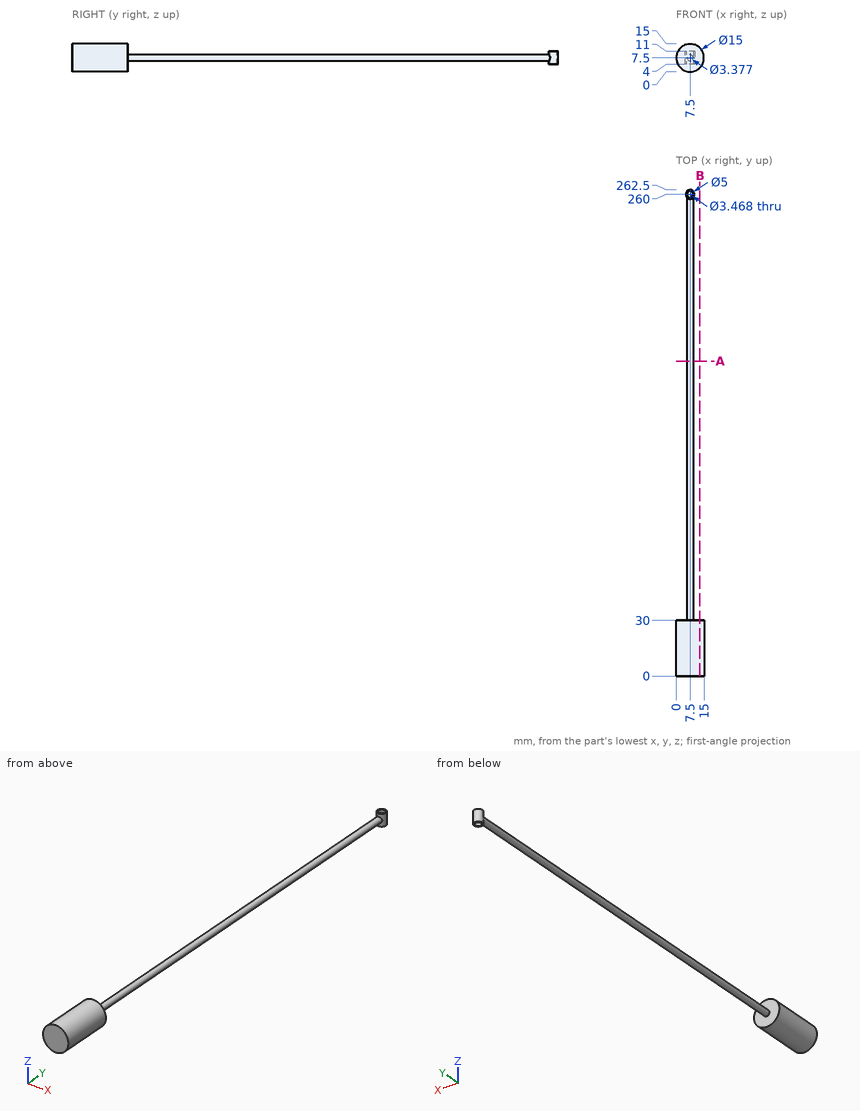
Here's the drawing with two shaded views (mm, measured from the low corner). I have some questions. Coordinates: 2 decimals unless noted, no trailing zeros. Write each loop counter-clockwise with the first axis right and the second up, starting at its lowest first coordinate (ties: lowest second). Pieces come first, ordered by that corner, then holes. Notation, with made-up numbers: M 56,40 L 79,40 A25 ccw 79,65 Z; hole C 73.5,79.5 d2. An arc over 180 degrees is marked long. Write item = value, one per line. Start each with the question number.
Q1. If we section it at B-B, the plane x = 12.75: Write out the boundary of the cut face in (y, z).
Q2. I'm going to push flat-ended pins straight in: pin 1 (1 mm diameter, centred on x = 9.5, y = 37, fed in from -Z) (1 decimal); pin 2 (6 mm diameter, centred on x = 6, y = 185, fed in from +Z); pin 3 (4 mm diameter, centred on x = 7.5, y = 260, fed in from +Z). Where does each tip first touch, or does it pass through?
Q3. If I drill on L1, parallel to X at y = 260, z = 7; L2, parallel to Y at x = 7.5, z = 6; L3, parallel to Y at x = 4.75, z = 5.75, over which ranges is the centre line in solid material (lowest first)? Write a range as [from, to].
Q4. If we section it at A-A, the plane y = 170: Write out the boundary of the cut face in (x, z).
Check sheet entries:
q1.outline = M 0,2.14 L 30,2.14 L 30,12.86 L 0,12.86 Z
q2.pin_1 = 6.7
q2.pin_2 = 9.19
q2.pin_3 = 11
q3.L1 = [5, 5.77], [9.23, 10]
q3.L2 = [0, 258.27], [261.73, 262.5]
q3.L3 = [0, 30]
q4.outline = C 7.5,7.5 d3.38
